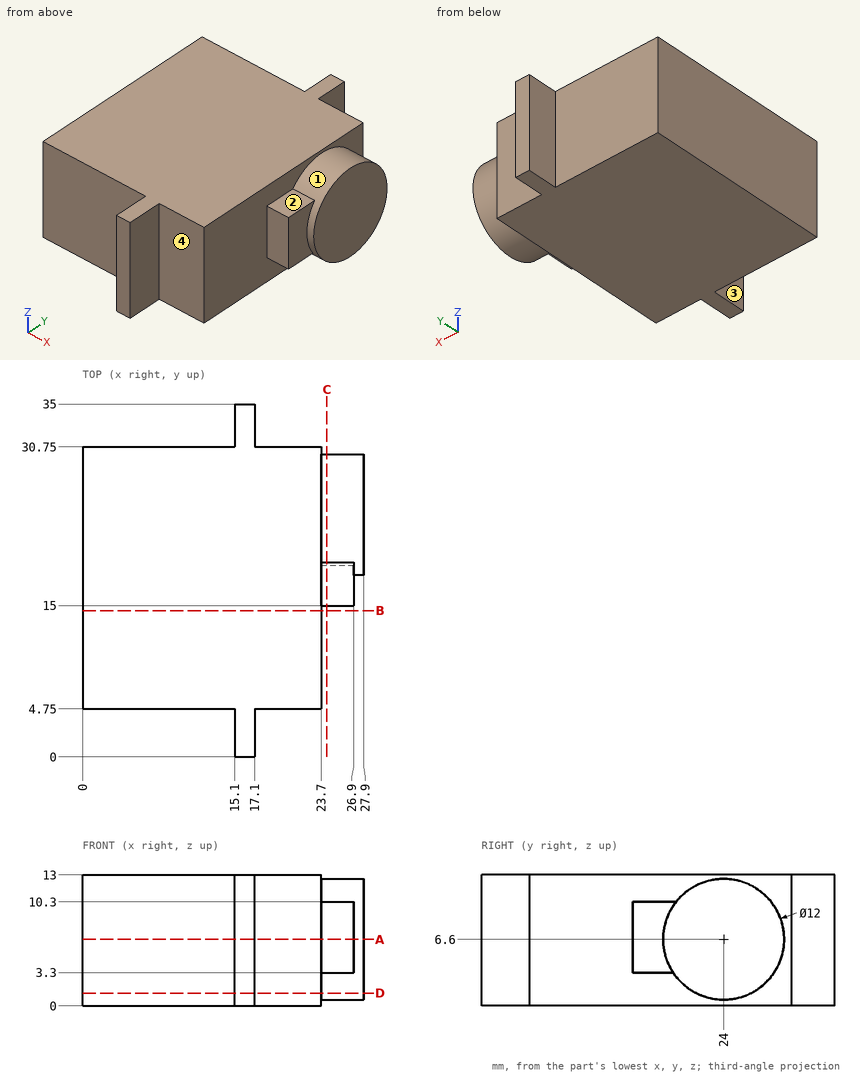
Geometry check sheet. Reference: drawing and pictorial views, mm from the part's lowest x, y, z. A direction names the side the tool comes from. Round coordinates to 2 decimals unless told otherwise and drop trailing zeros. Loops run counter-clockwise (first coordinate to the right, second up) from the corner with the lowest first, then second, coordinate; pieces in that order, holes last. Notation, with made-up numbers: (80.5, -23.5) - (122.5, -23.5) arc R20 cw to (122.5, -15.5) - close; hole circle Ø6 at (-20, 11). An arc over 180 degrees is marked (long way). One line per question, with ' | ' between items. Start each with the question number.
1. Cross-section at A-A on z = 6.6. Record the cut outline in (x, y), then the cut area to 3 significant figures.
2. Scan lines: line 1 (X direction, y = 4, z = 3.25); line 2 (X direction, y = 8.5, z = 10); line 3 (Y direction, x = 26, z = 6.5). Record each from-to range of solid material in increasing order. Write a range as [from, to].
3. Cross-section at D-D on z = 1.25. Record the cut outline in (x, y).
4. Depth check by flat-ended pin: pin 1 (6.5 mm diameter, centred on x = 10.5, z = 8, fed in from -Y); pin 2 (3.5 mm diameter, centred on x = 20, z = 3.5, fed in from +Y); pin 3 (1.3 mm diameter, centred on y = 32.5, z = 7, fed in from -X). Enter the tip coordinate at first touch or a pass-through.
5. Tool access check on the marked faces 1, 2, 3 and 4. Record the directions out of +Z, -Z, +X, -X, +Y, -Y that give a thin tool (end or side, any length) a straight path to the whole face; none if there is none.
6. Cross-section at B-B on y = 14.5. Record the cut outline in (x, z), then the cut area to 3 significant figures.
7. Cross-section at C-C on x = 24.25. Record the cut outline in (y, z).
Taken from the geometry:
1) outline: (0, 4.75) - (15.1, 4.75) - (15.1, 0) - (17.1, 0) - (17.1, 4.75) - (23.7, 4.75) - (23.7, 15) - (26.9, 15) - (26.9, 18) - (27.9, 18) - (27.9, 30) - (23.7, 30) - (23.7, 30.75) - (17.1, 30.75) - (17.1, 35) - (15.1, 35) - (15.1, 30.75) - (0, 30.75) - close | area: 694 mm²
2) line 1: [15.1, 17.1] | line 2: [0, 23.7] | line 3: [15, 30]
3) outline: (0, 4.75) - (15.1, 4.75) - (15.1, 0) - (17.1, 0) - (17.1, 4.75) - (23.7, 4.75) - (23.7, 21.28) - (27.9, 21.28) - (27.9, 26.72) - (23.7, 26.72) - (23.7, 30.75) - (17.1, 30.75) - (17.1, 35) - (15.1, 35) - (15.1, 30.75) - (0, 30.75) - close
4) pin 1: y = 4.75 | pin 2: y = 30.75 | pin 3: x = 15.1
5) face 1: +X | face 2: +Z, +X, -Y | face 3: +Z, -Z, -X, -Y | face 4: +Z, -Z, +X, -Y
6) outline: (0, 0) - (23.7, 0) - (23.7, 13) - (0, 13) - close | area: 308 mm²
7) outline: (15, 3.3) - (18.99, 3.3) arc R6 ccw (long way) to (19.28, 10.3) - (15, 10.3) - close
